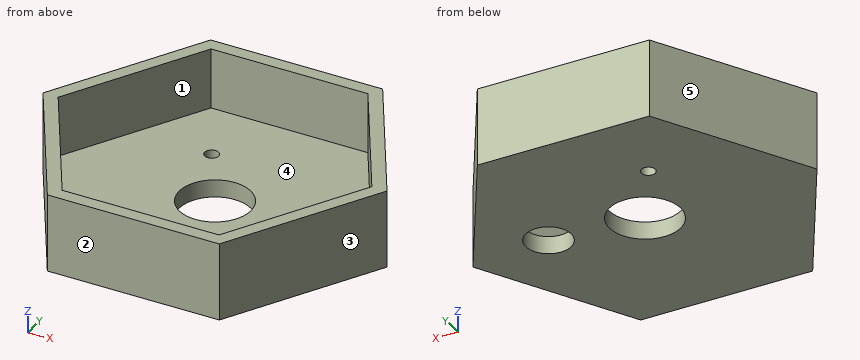
from build123d import *

# Parameters (mm, degrees)
F0_R     = 2.3
F0_R_2   = 11.75
F0_R_3   = 7.5
F1_DEPTH = 5.8
F2_DEPTH = 25.8


with BuildPart() as f1:
    # F0 (on Top) → F1 (new body)
    with BuildSketch(Plane.XY):
        Polygon((25.9, 44.860116), (-25.9, 44.860116), (-51.8, 0), (-25.9, -44.860116), (25.9, -44.860116), (51.8, 0), align=None)
        with Locations((-13.384125, 22.388888)):
            Circle(F0_R, mode=Mode.SUBTRACT)
        Circle(F0_R_2, mode=Mode.SUBTRACT)
        with Locations((30.454506, 2.57507)):
            Circle(F0_R_3, mode=Mode.SUBTRACT)
    extrude(amount=F1_DEPTH)

    # F0 (on Top) → F2 (join)
    with BuildSketch(Plane.XY):
        Polygon((28.4, 49.190243), (-28.4, 49.190243), (-56.8, 0), (-28.4, -49.190243), (28.4, -49.190243), (56.8, 0), align=None)
        Polygon((-51.8, 0), (-25.9, 44.860116), (25.9, 44.860116), (51.8, 0), (25.9, -44.860116), (-25.9, -44.860116), align=None, mode=Mode.SUBTRACT)
    extrude(amount=F2_DEPTH)


solid = f1.part
Read the model definition and answer for the solid it produces. Units are mm, in the model's axes. Face numbers are marked on the shaded views. A direction names the side the tool comes from. Coordinates: 2 decimals unless noted, no trailing zeros. Loops run counter-clockwise (first coordinate to the right, second up) from the corner with the lowest first, then second, coordinate; pieces in that order, holes last. Notation, with made-up numbers: (43, 82) - (66, 82) arc R12 cw to (66, 99) - close; hole circle Ø5 at (-24, 47.5). An arc over 180 degrees is marked (long way). Answer in a Markdown table with one row per item.
Q1. The mould has two halves that part along X. Classify the marked faces 3, 4 and 5: pulls with the +X half, pulls with the -X half, needs draft (parallel to the pull), parting line crosses it, or undercut.
Here are the results:
| item | result |
|---|---|
| face 3 | pulls with the +X half |
| face 4 | undercut |
| face 5 | pulls with the -X half |
Q2. Straight lines are drawn through the part: line 1 along Y through (x, z) = (23.5, 21.5); line 2 along Y through (x, z) = (0, 4.35); line 3 along Z through (x, y) = (-22.5, -4). For each, find the intervals that lie inside material, in ascending order. Write a range as [from, to].
Here are the results:
| item | result |
|---|---|
| line 1 | y = [-49.19, -44.86], [44.86, 49.19] |
| line 2 | y = [-49.19, -11.75], [11.75, 49.19] |
| line 3 | z = [0, 5.8] |
Q3. Find section A-A on x = 0. Write down the section's boundary in (y, z).
Here are the results:
| item | result |
|---|---|
| outline | (-49.19, 0) - (-11.75, 0) - (-11.75, 5.8) - (-44.86, 5.8) - (-44.86, 25.8) - (-49.19, 25.8) - close; (11.75, 0) - (49.19, 0) - (49.19, 25.8) - (44.86, 25.8) - (44.86, 5.8) - (11.75, 5.8) - close |
Q4. Find section D-D on y = -9. Write down the section's boundary in (x, z), plus the area to 3 significant figures.
Here are the results:
| item | result |
|---|---|
| outline | (-51.6, 0) - (-7.55, 0) - (-7.55, 5.8) - (-46.6, 5.8) - (-46.6, 25.8) - (-51.6, 25.8) - close; (7.55, 0) - (51.6, 0) - (51.6, 25.8) - (46.6, 25.8) - (46.6, 5.8) - (7.55, 5.8) - close |
| area | 711 mm^2 |
Q5. Given P1, Ø6, axis at y = -10.5, z = 10, coming from the -X side; P2, Ø4, axis at y = -19.5, z = 9.5, coming from the -X side; P3, Ø1, axis at x = -10, y = -39.5, coming from the +Z side, each flat-ended and moving along its own axis, determine where each tip first touches the part or whether it passes through.
Here are the results:
| item | result |
|---|---|
| P1 | stops at x = -52.47 |
| P2 | stops at x = -46.7 |
| P3 | stops at z = 5.8 |
Q6. For the marked faces 1 and 2, determine the directions among +Z, -Z, +X, -X, +Y, -Y from which every point of the face is accessible in a straight line to the end or side of a thin tool.
Here are the results:
| item | result |
|---|---|
| face 1 | +Z |
| face 2 | +Z, -Z, +X, -X, -Y |
Q7. Find section B-B on z = 23. Write down the section's boundary in (x, y), plus the area to 3 significant figures.
Here are the results:
| item | result |
|---|---|
| outline | (-56.8, 0) - (-28.4, -49.19) - (28.4, -49.19) - (56.8, 0) - (28.4, 49.19) - (-28.4, 49.19) - close; hole (-51.8, 0) - (-25.9, -44.86) - (25.9, -44.86) - (51.8, 0) - (25.9, 44.86) - (-25.9, 44.86) - close |
| area | 1,410 mm^2 |
Q8. Find section C-C on x = 19.5. Write down the section's boundary in (y, z), plus the area to 3 significant figures.
Here are the results:
| item | result |
|---|---|
| outline | (-49.19, 0) - (49.19, 0) - (49.19, 25.8) - (44.86, 25.8) - (44.86, 5.8) - (-44.86, 5.8) - (-44.86, 25.8) - (-49.19, 25.8) - close |
| area | 744 mm^2 |
